Read the model definition and answer for the solid it produces. Units are mm, in the model's axes. A direction names the side the tool comes from. Give positions to 0.01 mm unless a question says otherwise; leave off trailing zeros. Write each loop counter-clockwise with the first axis right and the second up, starting at its lowest first coordinate (ties: lowest second). Pieces come first, ordered by that corner, then holes. Notation, with made-up numbers: M -10.5,69 L 0.5,69 A31 ccw 0.5,100 Z; hole C -25.75,-10 d4. An arc over 180 degrees is marked long. Use a Markdown table: item, result. Add a question column.
Item 1: A cutting plane is placed at A-A on x = 0. Determine the outline of the cut face in (y, z), then the cut area to 3 significant figures.
Item 2: The mould has two halves that part along Z. Classify faces 1 (the flat face through (0, 4.442, 5)), 2 (the cylindrical face through (-16.147, 2.209, 13.953)), 3 (the flat face through (-8.94, -0.61, 13.78)), 4 (the cylindrical face through (-0.22, -0.49, 7.42)): pulls with the +Z half, pulls with the -Z half, needs draft (parallel to the pull), parting line crosses it, or undercut.
Item 3: Consider probe 1 along Z at (x, y) = (0, -3); probe 2 along Y at (x, z) = (-12.75, 11.5); probe 3 along Z at (x, y) = (0, -2). Determine where each line is inside the solid, lowest interval first. Write a range as [from, to].
Item 4: A cutting plane is placed at D-D on z = 9. Determine the outline of the cut face in (x, y).
Item 5: A cutting plane is placed at B-B on y = 0. Determine the outline of the cut face in (x, z).
Item 6: Given P1, Ø3, axis at x = -15.41, z = 14.63, coming from the -Y side; P2, Ø5.5, axis at x = -13, z = 13.5, coming from the +Y side; P3, Ø2, axis at x = -11.5, y = -0.5, coming from the -Z side, each flat-ended and moving along its own axis, determine where each tip first touches the part or whether it passes through.
Item 7: A cutting plane is placed at C-C on y = -3.5. Determine the outline of the cut face in (x, z) (1 decimal).
Item 8: For faces 5 (the flat face through (-11.13, -0.61, 9.27)), 6 (the cylindrical face through (-0.867, -3.905, 1.315)), 7 (the flat face through (0, -5.558, 5)), 8 (the cylindrical face through (4.6, -0.5, 8.4)), 9 (the flat face through (-13.316, -0.579, 13.38)), determine the directions among +Z, -Z, +X, -X, +Y, -Y from which every point of the face is accessible in a straight line to the end or side of a thin tool.
from build123d import *

# Parameters (mm, degrees)
SKETCH2_R                       = 4
SKETCH2_R_2                     = 2.5
BOSS_EXTRUDE1_DEPTH             = 4
SKETCH4_R                       = 5
BOSS_EXTRUDE2_DEPTH             = 10
SKETCH5_R                       = 2.5
CUT_EXTRUDE1_DEPTH              = 5
SKETCH6_R                       = 1
CUT_EXTRUDE2_DEPTH              = 11.0000001
SKETCH7_W                       = 8
SKETCH7_H                       = 5
BOSS_EXTRUDE3_DEPTH             = 15
BOSS_EXTRUDE3_DIRECTION_2_REACH = 14.552
SKETCH10_W                      = 5
SKETCH10_H                      = 3
CUT_EXTRUDE4_DEPTH              = 20
SKETCH9_R                       = 1
CUT_EXTRUDE6_DEPTH              = 20


with BuildPart() as part:
    # Sketch2 → Boss-Extrude1 (new body)
    with BuildSketch(Plane.XY):
        Circle(SKETCH2_R)
        Circle(SKETCH2_R_2, mode=Mode.SUBTRACT)
    extrude(amount=BOSS_EXTRUDE1_DEPTH)

    # Sketch4 → Boss-Extrude2 (add)
    with BuildSketch(Plane(origin=(0, 4.441770998, 4), x_dir=(1, 0, 0), z_dir=(0, 1, 0))):
        with Locations((0, -2.444351266)):
            Circle(SKETCH4_R)
    extrude(amount=-BOSS_EXTRUDE2_DEPTH)

    # Sketch5 → Cut-Extrude1 (cut)
    with BuildSketch(Plane.XY):
        Circle(SKETCH5_R)
    extrude(amount=CUT_EXTRUDE1_DEPTH, mode=Mode.SUBTRACT)

    # Sketch6 → Cut-Extrude2 (cut, through all)
    with BuildSketch(Plane(origin=(0, 4.441770998, 0), x_dir=(1, 0, 0), z_dir=(0, 1, 0))):
        with Locations((0, -6.444351266)):
            Circle(SKETCH6_R)
    extrude(amount=-CUT_EXTRUDE2_DEPTH, mode=Mode.SUBTRACT)

    # Sketch7 → Boss-Extrude3 (add)
    with BuildSketch(Plane(origin=(-7.120612972, 0, 4.111087816), x_dir=(0, 1, 0), z_dir=(-0.866025404, 0, 0.5))):
        with Locations((-0.558229002, -4.964101615)):
            Rectangle(SKETCH7_W, SKETCH7_H)
    extrude(amount=BOSS_EXTRUDE3_DEPTH)

    # Sketch7 → Boss-Extrude3 direction 2 (add, up to next)
    with BuildSketch(Plane(origin=(-7.120612972, 0, 4.111087816), x_dir=(0, 1, 0), z_dir=(-0.866025404, 0, 0.5)), mode=Mode.PRIVATE) as boss_extrude3_direction_2_sk1:
        with Locations((-0.558229002, -4.964101615)):
            Rectangle(SKETCH7_W, SKETCH7_H)
    boss_extrude3_direction_2_tool1 = extrude(boss_extrude3_direction_2_sk1.sketch, amount=-BOSS_EXTRUDE3_DIRECTION_2_REACH, mode=Mode.PRIVATE) - part.part
    add(boss_extrude3_direction_2_tool1.solids().sort_by_distance((-4.638562, -0.558229, 8.410126))[0])
    add(boss_extrude3_direction_2_tool1.solids().sort_by_distance((-4.638562, -0.558229, 8.410126))[1])

    # Sketch10 → Cut-Extrude4 (cut)
    with BuildSketch(Plane(origin=(1.232050808, 0, 2.133974596), x_dir=(-0.866025404, 0, 0.5), z_dir=(-0.5, 0, -0.866025404))):
        with Locations((20.722175633, -0.558229002)):
            Rectangle(SKETCH10_W, SKETCH10_H)
    extrude(amount=-CUT_EXTRUDE4_DEPTH, mode=Mode.SUBTRACT)

    # Sketch9 → Cut-Extrude6 (cut)
    with BuildSketch(Plane(origin=(0, 3.441770998, 0), x_dir=(1, 0, 0), z_dir=(0, 1, 0))):
        with BuildLine():
            Line((-18.878943222, -13.745062413), (-17.628943256, -15.910125863))
            ThreePointArc((-17.628943256, -15.910125863), (-17.943039978, -14.243046987), (-17.146892414, -12.745062413))
            Line((-17.146892414, -12.745062413), (-18.878943222, -13.745062413))
        make_face()
        with BuildLine():
            Line((-17.628943256, -15.910125863), (-16.378943222, -18.075189432))
            Line((-16.378943222, -18.075189432), (-14.646892414, -17.075189432))
            ThreePointArc((-14.646892414, -17.075189432), (-16.342258956, -17.015681135), (-17.628943256, -15.910125863))
        make_face()
        with Locations((-15.409753124, -14.628875922)):
            Circle(SKETCH9_R)
    extrude(amount=-CUT_EXTRUDE6_DEPTH, mode=Mode.SUBTRACT)


solid = part.part
Filled in:
| question | item | result |
|---|---|---|
| 1 | outline | M -5.56,1.44 L -4,1.44 L -4,0 L -2.5,0 L -2.5,5 L 2.5,5 L 2.5,0 L 4,0 L 4,1.44 L 4.44,1.44 L 4.44,5.44 L -5.56,5.44 Z; M -5.56,7.44 L 4.44,7.44 L 4.44,11.44 L -5.56,11.44 Z |
| 1 | area | 66.6 mm² |
| 2 | face 1 | needs draft |
| 2 | face 2 | undercut |
| 2 | face 3 | pulls with the +Z half |
| 2 | face 4 | undercut |
| 3 | probe 1 | [0, 5.44], [7.44, 11.44] |
| 3 | probe 2 | [-4.56, 3.44] |
| 3 | probe 3 | [5, 5.44], [7.44, 11.44] |
| 4 | outline | M -10.66,-4.56 L -4.3,-4.56 L -4.3,-5.56 L 4.3,-5.56 L 4.3,4.44 L -4.3,4.44 L -4.3,3.44 L -10.66,3.44 Z |
| 5 | outline | M -14.55,11.25 L -4.94,5.7 A5 ccw -4,3.44 L -4,0 L -2.5,0 L -2.5,5 L 2.5,5 L 2.5,0 L 4,0 L 4,3.44 A5 ccw -3.07,10.39 L -12.05,15.58 Z; hole C 0,6.44 d2 |
| 6 | P1 | y = -4.56 |
| 6 | P2 | y = 3.44 |
| 6 | P3 | z = 8.91 |
| 7 | outline | M -17.1,12.7 L -4.9,5.7 A5 ccw -1.9,1.8 L -1.9,0 L 1.9,0 L 1.9,1.8 A5 ccw long -3.1,10.4 L -14.6,17.1 A2.6 ccw Z; hole C -15.4,14.6 d2; hole C 0,6.4 d2 |
| 8 | face 5 | -Z, -X, +Y, -Y |
| 8 | face 6 | -Z |
| 8 | face 7 | +Z, -Z, +X, -X, -Y |
| 8 | face 8 | none |
| 8 | face 9 | +Z, -X |
